```python
from build123d import *

# Parameters (mm, degrees)
F0_W     = 199.2195397615
F0_H     = 111.6918176413
F1_DEPTH = 75
F2_W     = 199.2195397615
F2_H     = 55.8459088206
F3_DEPTH = 59.6
F4_W     = 173.3557134867
F4_H     = 32.2399325669
F5_DEPTH = 59.9
F6_R     = 5


with BuildPart() as f1:
    # F0 (on Front) → F1 (new body)
    with BuildSketch(Plane.XZ):
        Rectangle(F0_W, F0_H)
    extrude(amount=F1_DEPTH)

    # F2 (on face) → F3 (cut)
    with BuildSketch(Plane.XZ.offset(75)):
        with Locations((0, 27.9229544103)):
            Rectangle(F2_W, F2_H)
    extrude(amount=-F3_DEPTH, mode=Mode.SUBTRACT)

    # F4 (on face) → F5 (cut)
    with BuildSketch(Plane.XZ.offset(75)):
        with Locations((-0.2642646432, -16.1199662834)):
            Rectangle(F4_W, F4_H)
    extrude(amount=-F5_DEPTH, mode=Mode.SUBTRACT)

    # F6
    f6_edges = [f1.edges().sort_by_distance(p)[0] for p in [
        (-99.60977, -45.2, 0),
        (-86.942121, -45.2, 0),
        (-86.942121, -45.05, -32.239933),
        (86.413592, -45.05, -32.239933),
        (86.413592, -45.2, 0),
        (99.60977, -45.2, 0),
        (-99.60977, -15.4, 27.922954),
        (0, -15.4, 55.845909),
        (99.60977, -15.4, 27.922954),
    ]]
    fillet(f6_edges, radius=F6_R)


solid = f1.part
```
The listing builds one solid part. Answer for the finished solid, in the listing's coordinates (mm). A direction names the side the tool comes from. Give positions to 0.01 mm unless a question says otherwise; leave off trailing zeros. Order: outer loops, then holes, each group sorted by start corner. A loop starts at its lowest first (then second) coordinate and runs counter-clockwise, first axis right, second up.
Item 1: Given pin 1 Ø6 at (x, y) = (28, -66) entering from +Z; pin 2 Ø16 at (x, z) = (11.5, -23) entering from -Y; pin 3 Ø1 at (x, y) = (93.5, -49) entering from +Z; pin 4 Ø5 at (x, z) = (1.5, 2) entering from +Y, each flat-ended and moving along its own axis, determine where each tip first touches the part or whether it passes through.
From the geometry:
pin 1: stops at z = -32.24
pin 2: stops at y = -15.1
pin 3: stops at z = 0
pin 4: stops at y = 0
Item 2: Find the intervals of material crossed by probe 1 along X at (y, z) = (-48, -11.5); probe 2 along Y at (x, z) = (49.5, -13); probe 3 along Z at (x, y) = (-92, -37.5), in increasing order.
From the geometry:
probe 1: x = -99.61 to -86.94, 86.41 to 99.61
probe 2: y = -15.1 to 0
probe 3: z = -55.85 to 0
Item 3: For a pull along X with two mould halves and no side action, classify faces 6 (the face through (-1, -15.1, -16)), 7 (the face through (98.11, -13.97, 25.85)), 8 (the face through (-1, -75, -40)) as pulls with the +X half, pulls with the -X half, needs draft (parallel to the pull), parting line crosses it, or undercut.
From the geometry:
face 6: undercut
face 7: pulls with the +X half
face 8: needs draft
Item 4: The part is cut by section A-A, the plane z = 29.5. Give the vertices of the cut face in (x, y).
From the geometry:
outline: (-99.61, -10.4) arc R5 ccw to (-94.61, -15.4) - (94.61, -15.4) arc R5 ccw to (99.61, -10.4) - (99.61, 0) - (-99.61, 0) - close
Item 5: The part is cut by section C-C, the plane x = 16. Give the vertices of the cut face in (y, z).
From the geometry:
outline: (-75, -55.85) - (0, -55.85) - (0, 55.85) - (-10.4, 55.85) arc R5 ccw to (-15.4, 50.85) - (-15.4, 0) - (-15.1, 0) - (-15.1, -32.24) - (-75, -32.24) - close
Item 6: The part is cut by section B-B, the plane y = -38.5. Give the vertices of the cut face in (x, z), and give its area (3 significant figures).
From the geometry:
outline: (-99.61, -55.85) - (99.61, -55.85) - (99.61, -5) arc R5 ccw to (94.61, 0) - (91.41, 0) arc R5 ccw to (86.41, -5) - (86.41, -27.24) arc R5 cw to (81.41, -32.24) - (-81.94, -32.24) arc R5 cw to (-86.94, -27.24) - (-86.94, -5) arc R5 ccw to (-91.94, 0) - (-94.61, 0) arc R5 ccw to (-99.61, -5) - close
area: 5,530 mm2
Item 7: Which of the six approach directions +Z, -Z, +X, -X, +Y, -Y give full straight-line access (tool end or side, diameter ignored) to faces 1 (the face through (99.61, -37, -26)), 2 (the face through (84.91, -44.631, -30.814)), 3 (the face through (-1, -5, 55.846)), 4 (the face through (98.18, -42.25, -1.5)), 5 (the face through (-98.18, -42.25, -1.5))?
From the geometry:
face 1: +Z, -Z, +X, +Y, -Y
face 2: +Z, -Y
face 3: +Z, +X, -X, +Y, -Y
face 4: +Z, +X, -Y
face 5: +Z, -X, -Y
Item 8: The part is cut by section D-D, the plane z = -19. Give the vertices of the cut face in (x, y).
From the geometry:
outline: (-99.61, -75) - (-86.94, -75) - (-86.94, -15.1) - (86.41, -15.1) - (86.41, -75) - (99.61, -75) - (99.61, 0) - (-99.61, 0) - close
